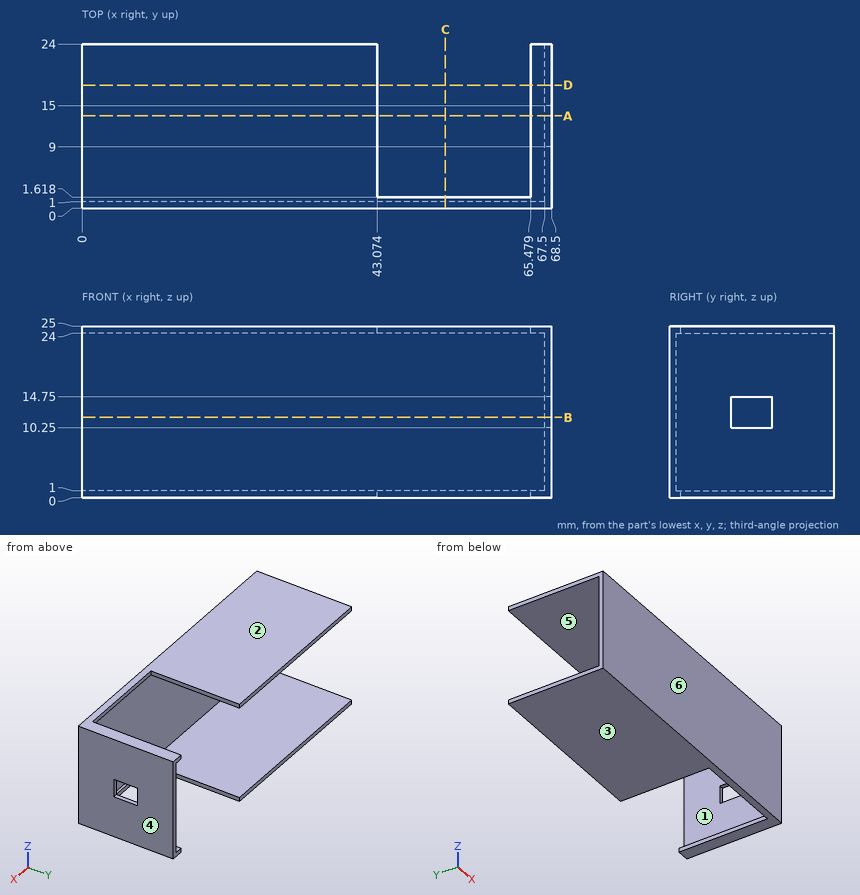
Part print with two shaded views. Sizes in mm from the minimum x, y, z corner. A direction names the side the tool comes from. Coordinates: 2 decimals unless noted, no trailing zeros. Loops run counter-clockwise (first coordinate to the right, second up) from the corner with the lowest first, then second, coordinate; pieces in that order, holes last. Notation, with made-up numbers: (51.25, 22.5) - (93.25, 22.5) arc R22 cw to (93.25, 39.5) - close; hole circle Ø3 at (8, 27.25). An arc over 180 degrees is marked (long way). Write each question's results on one line, items separated by ' | '. Start each with the question number.
Q1. Slice it at C-C on x = 53. Give the cut face in (y, z).
Q2. Slice it at D-D on y = 18. Give the cut face in (x, z), and give its area (3 significant figures).
Q3. Which spindle directions (+Z, -Z, +X, -X, +Y, -Y) get a long thin tool onto all of the face, cutting with end or side? Do the marked faces 5 and 6. Say none if no direction does.
Q4. Drop flat-ended pins along their axis: pin 1 Ø10 at (x, y) = (12.5, 2.5) entering from -Z; pin 2 Ø6 at (y, z) = (15.5, 4.5) entering from -X; pin 3 Ø11.5 at (x, z) = (43, 9.5) entering from +Y. Give the stop position or say it passes through.
Q5. Two-plate mould, pull along Z, no slides. Class the marked faces 1, 2, 3 and 4: +Z half, -Z half, draft (parallel to the pull), parting line (faces both ways), or undercut.
Q6. Slice it at B-B on z = 11.75. Give the cut face in (x, y).
Q7. Slice it at A-A on y = 13.5. Give the cut face in (x, z).
Q8. Probe line 1 along Z through (x, y) = (9.5, 7.5); line 2 along X through (y, z) = (5.75, 8); line 3 along Y through (x, z) = (18.5, 23.75). List the from-to ranges inside material, lowest first.
Answer:
1) outline: (0, 0) - (1.62, 0) - (1.62, 1) - (1, 1) - (1, 24) - (1.62, 24) - (1.62, 25) - (0, 25) - close
2) outline: (0, 0) - (43.07, 0) - (43.07, 1) - (0, 1) - close; (0, 24) - (43.07, 24) - (43.07, 25) - (0, 25) - close; (65.48, 0) - (68.5, 0) - (68.5, 25) - (65.48, 25) - (65.48, 24) - (67.5, 24) - (67.5, 1) - (65.48, 1) - close | area: 115 mm2
3) face 5: -X, +Y | face 6: +Z, -Z, +X, -X, -Y
4) pin 1: stops at z = 0 | pin 2: stops at x = 67.5 | pin 3: stops at y = 1
5) face 1: undercut | face 2: +Z half | face 3: -Z half | face 4: draft
6) outline: (0, 0) - (68.5, 0) - (68.5, 9) - (67.5, 9) - (67.5, 1) - (0, 1) - close; (67.5, 15) - (68.5, 15) - (68.5, 24) - (67.5, 24) - close
7) outline: (0, 0) - (43.07, 0) - (43.07, 1) - (0, 1) - close; (0, 24) - (43.07, 24) - (43.07, 25) - (0, 25) - close; (65.48, 0) - (68.5, 0) - (68.5, 10.25) - (67.5, 10.25) - (67.5, 1) - (65.48, 1) - close; (65.48, 24) - (67.5, 24) - (67.5, 14.75) - (68.5, 14.75) - (68.5, 25) - (65.48, 25) - close
8) line 1: z = 0 to 1, 24 to 25 | line 2: x = 67.5 to 68.5 | line 3: y = 0 to 1
